The model under review builds one solid part; all positions refer to its coordinate system, in mm. A direction names the side the tool comes from. Round coordinates to 2 decimals unless told otherwise and drop trailing zeros. Order: outer loops, then holes, each group sorted by start corner. A loop starts at its lowest first (then second) coordinate and runs counter-clockwise, first axis right, second up.
```python
from build123d import *

# Parameters (mm, degrees)
SKETCH1_W                   = 146.05
SKETCH1_H                   = 101.6
SKETCH1_R                   = 1.75
SKETCH1_W_2                 = 28
SKETCH1_H_2                 = 50
BOSS_EXTRUDE1_DEPTH         = 4
F_1_4_CLEARANCE_HOLE1_D     = 6.7564
F_1_4_CLEARANCE_HOLE1_DEPTH = 12
F_1_4_CLEARANCE_HOLE1_TIP   = 2.029827343
CHAMFER1_SIZE               = 2


with BuildPart() as part:
    # Sketch1 → Boss-Extrude1 (new body)
    with BuildSketch(Plane.XY):
        Rectangle(SKETCH1_W, SKETCH1_H)
        with Locations((-19.75, 0)):
            Circle(SKETCH1_R, mode=Mode.SUBTRACT)
        with Locations((19.75, 0)):
            Circle(SKETCH1_R, mode=Mode.SUBTRACT)
        Rectangle(SKETCH1_W_2, SKETCH1_H_2, mode=Mode.SUBTRACT)
    extrude(amount=BOSS_EXTRUDE1_DEPTH)

    # 1/4 Clearance Hole1
    with Locations(Plane.XY.offset(4)):
        with Locations((-53.975, 38.1), (53.975, 38.1), (53.975, -38.1), (-53.975, -38.1)):
            Hole(F_1_4_CLEARANCE_HOLE1_D / 2, depth=F_1_4_CLEARANCE_HOLE1_DEPTH)
            with Locations((0, 0, -(F_1_4_CLEARANCE_HOLE1_DEPTH + F_1_4_CLEARANCE_HOLE1_TIP / 2))):  # 118° drill point
                Cone(0, F_1_4_CLEARANCE_HOLE1_D / 2, F_1_4_CLEARANCE_HOLE1_TIP, mode=Mode.SUBTRACT)

    # Chamfer1
    chamfer1_edges = [part.edges().sort_by_distance(p)[0] for p in [
        (-73.025, -50.8, 2),
        (-73.025, 50.8, 2),
        (73.025, 50.8, 2),
        (73.025, -50.8, 2),
    ]]
    chamfer(chamfer1_edges, length=CHAMFER1_SIZE)


solid = part.part
```
(1) Consider section D-D (y = -38.1). Write out the cut boundary in (x, z) (3 decimals), and give its area (3 significant figures).
Data:
outline: (-73.025, 0) - (-57.353, 0) - (-57.353, 4) - (-73.025, 4) - close; (-50.597, 0) - (50.597, 0) - (50.597, 4) - (-50.597, 4) - close; (57.353, 0) - (73.025, 0) - (73.025, 4) - (57.353, 4) - close
area: 530 mm2
(2) For faces 1 (the flat face through (-14, 0, 2)), 2 (the flat face through (-1, -50.8, 2)), list the 3-axis set-ups (+Z, -Z, +X, -X, +Y, -Y) from which the entire face can be reached by the end or side of a thin tool; tool diameter is ignored.
Data:
face 1: +Z, -Z
face 2: +Z, -Z, +X, -X, -Y
(3) To check wall thickness, follow probe 1 along X at (y, z) = (20, 2.8) (3 decimals); probe 2 along Y at (x, z) = (55, 2.4); probe 3 along Y at (x, z) = (-19.75, 2.25). State the ranges of each line that lie inside material, in increasing order.
Data:
probe 1: x = -73.025 to -14, 14 to 73.025
probe 2: y = -50.8 to -41.32, -34.88 to 34.88, 41.32 to 50.8
probe 3: y = -50.8 to -1.75, 1.75 to 50.8
(4) Consider section B-B (z = 2.4). Write out the cut boundary in (x, y) (3 decimals), and give its area (3 significant figures).
Data:
outline: (-73.025, -48.8) - (-71.025, -50.8) - (71.025, -50.8) - (73.025, -48.8) - (73.025, 48.8) - (71.025, 50.8) - (-71.025, 50.8) - (-73.025, 48.8) - close; hole circle Ø6.756 at (-53.975, -38.1); hole circle Ø6.756 at (-53.975, 38.1); hole circle Ø3.5 at (-19.75, 0); hole (-14, -25) - (14, -25) - (14, 25) - (-14, 25) - close; hole circle Ø3.5 at (19.75, 0); hole circle Ø6.756 at (53.975, -38.1); hole circle Ø6.756 at (53.975, 38.1)
area: 13,300 mm2
(5) Insertion check: pin 1 (6 mm diameter, centred on x = 53.975, y = 38.1, fed in from +Z). The pin has a flat end and moves straight along its axis. Give the tip position at first contact, or say it passes through.
Data:
pin 1: passes through
(6) Consider section A-A (y = 12.5). Write out the cut boundary in (x, z) (3 decimals), and give its area (3 significant figures).
Data:
outline: (-73.025, 0) - (-14, 0) - (-14, 4) - (-73.025, 4) - close; (14, 0) - (73.025, 0) - (73.025, 4) - (14, 4) - close
area: 472 mm2
(7) Consider section C-C (x = -19.75). Write out the cut boundary in (y, z), and give its area (3 significant figures).
Data:
outline: (-50.8, 0) - (-1.75, 0) - (-1.75, 4) - (-50.8, 4) - close; (1.75, 0) - (50.8, 0) - (50.8, 4) - (1.75, 4) - close
area: 392 mm2
(8) Draft analysis for pull direction X (two halves, no side actions). For faces 3 (the flat face through (0, 25, 2)), 4 (the flat face through (-17, 1, 4)), 5 (the cylindrical face through (18, 0, 2)), 6 (the flat face through (-73.025, -1, 2)), state which applies: pulls with the +X half, pulls with the -X half, needs draft (parallel to the pull), parting line crosses it, or undercut.
Data:
face 3: undercut
face 4: needs draft
face 5: undercut
face 6: pulls with the -X half
